Check sheet for the drawn part. Datum: minimum x, y, z corner. Units: mm. A direction names the side the tool comes from. Give positions to 0.01 mm unless a question says otherwise; leave off trailing zeros. Write each loop counter-clockwise with the first axis right and the second up, starting at its lowest first coordinate (ties: lowest second). Pieces come first, ordered by that corner, then holes. Notation, with made-up numbers: M 39.25,44.25 L 81.25,44.25 A12 cw 81.25,52.25 Z; hole C -18.5,20 d3. An arc over 180 degrees is marked long. Use CSV: the item, a comma, the result in double quotes. Start each with the question number.
1. Access from +Z, -Z, +X, -X, +Y, -Y to the whole of each face (thin tool, end or side, straight path). Record for the marked faces 4 and 5.
2. Mould release check, pull along Y, two halves, no side actions. Record for the marked faces 1, 2 and 3: +Y half, -Y half, draft (parallel to the pull), parting line (faces both ways), or undercut.
3. Depth check by flat-ended pin: P1, Ø8, axis at x = 648.5, y = 1015.5, coming from the -Z side. Enter the tip coordinate at first touch or a pass-through.
4. Cross-section at C-C, the plane z = 113. Enter the section's corners in (x, y), and give its area (3 significant figures).
5. Cross-section at A-A, the plane y = 1812.5. Enter the section's corners in (x, z).
6. Cross-section at B-B, the plane x = 389.5. Enter the section's corners in (y, z).
7. Scan lines: line 1 (X direction, y = 1298.5, z = 127.5); line 2 (Y direction, x = 298.5, z = 67.5); line 3 (Y direction, x = 265, z = 133). Record each from-to range of solid material in increasing order.
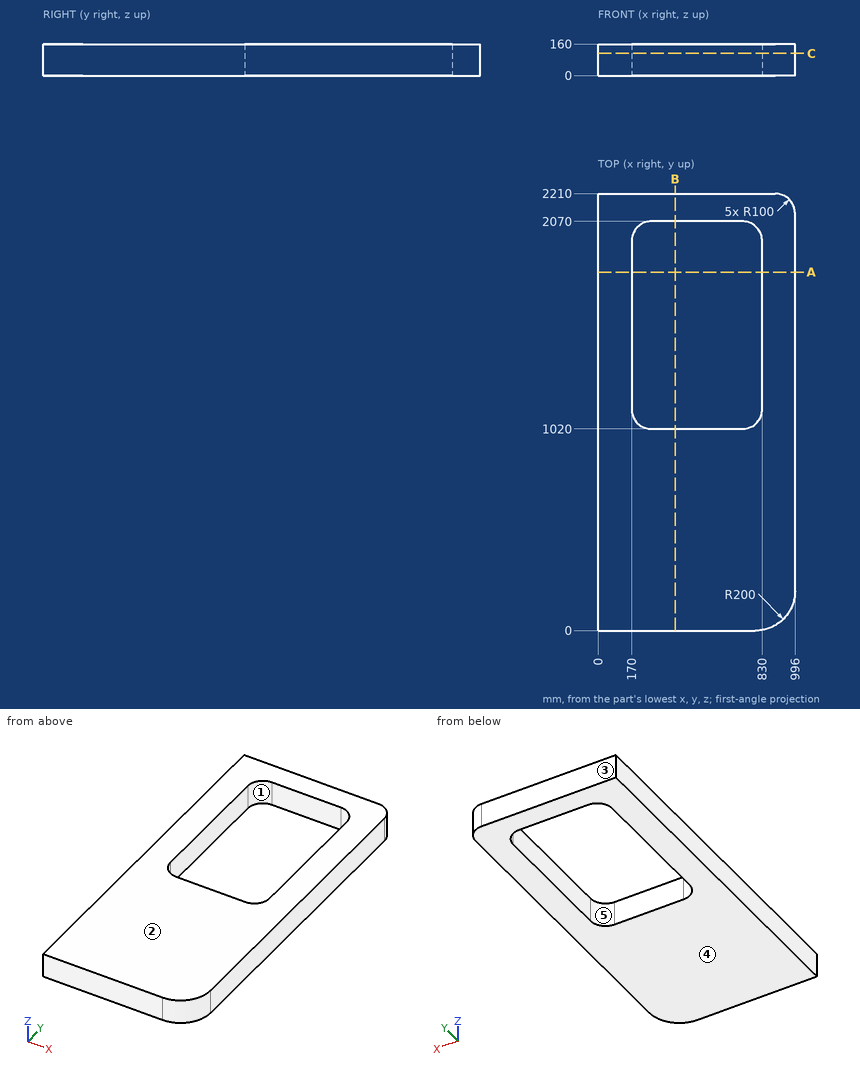
Worked answers:
1,face 4,"-Z, +X, -X, +Y, -Y"
1,face 5,"+Z, -Z"
2,face 1,"undercut"
2,face 2,"draft"
2,face 3,"+Y half"
3,P1,"stops at z = 0"
4,outline,"M 0,0 L 796,0 A200 ccw 996,200 L 996,2110 A100 ccw 896,2210 L 0,2210 Z; hole M 170,1120 A100 ccw 270,1020 L 730,1020 A100 ccw 830,1120 L 830,1970 A100 ccw 730,2070 L 270,2070 A100 ccw 170,1970 Z"
4,area,"1,510,000 mm^2"
5,outline,"M 0,0 L 170,0 L 170,160 L 0,160 Z; M 830,0 L 996,0 L 996,160 L 830,160 Z"
6,outline,"M 0,0 L 1020,0 L 1020,160 L 0,160 Z; M 2070,0 L 2210,0 L 2210,160 L 2070,160 Z"
7,line 1,"x = 0 to 170, 830 to 996"
7,line 2,"y = 0 to 1020, 2070 to 2210"
7,line 3,"y = 0 to 1020.13, 2069.87 to 2210"
